```python
from build123d import *

# Parameters (mm, degrees)
BOSS_EXTRUDE1_DEPTH            = 4.4
BOSS_EXTRUDE2_START            = 4.4
BOSS_EXTRUDE2_DEPTH            = 40
BOSS_EXTRUDE3_START            = 4.4
BOSS_EXTRUDE3_DEPTH            = 3
CUT_EXTRUDE1_START             = -37
CUT_EXTRUDE1_DEPTH             = 37
CUT_EXTRUDE2_DEPTH             = 120.718001988
CUT_EXTRUDE2_DEPTH_BACK        = 120.718001988
FILLET1_R                      = 10
CUT_EXTRUDE3_REACH             = 121.718
CUT_EXTRUDE3_DIRECTION_2_REACH = 121.718
FILLET2_R                      = 1
CHAMFER1_SIZE                  = 5
CUT_EXTRUDE4_REACH             = 141.367
CUT_EXTRUDE4_END_RADIUS        = 65


with BuildPart() as part:
    # Sketch1 → Boss-Extrude1 (new body)
    with BuildSketch(Plane(origin=(0, 0, 0), x_dir=(1, 0, 0), z_dir=(0, 1, 0))):
        with BuildLine():
            Line((-31.320919527, 25.2), (31.320919527, 25.2))
            Line((31.320919527, 25.2), (51.0779796, 40.2))
            ThreePointArc((51.0779796, 40.2), (-65, 0), (51.0779796, -40.2))
            Line((51.0779796, -40.2), (31.320919527, -25.2))
            Line((31.320919527, -25.2), (-31.320919527, -25.2))
            ThreePointArc((-31.320919527, -25.2), (-40.2, 0), (-31.320919527, 25.2))
        make_face()
    extrude(amount=BOSS_EXTRUDE1_DEPTH)

    # Sketch1<3> → Boss-Extrude2 (add)
    with BuildSketch(Plane(origin=(0, 0, 0), x_dir=(1, 0, 0), z_dir=(0, 1, 0)).offset(BOSS_EXTRUDE2_START)):
        with BuildLine():
            ThreePointArc((0, -55), (-55, 0), (0, 55))
            Line((0, 55), (34.641016151, 55))
            ThreePointArc((34.641016151, 55), (-65, 0), (34.641016151, -55))
            Line((34.641016151, -55), (0, -55))
        make_face()
    extrude(amount=BOSS_EXTRUDE2_DEPTH)

    # Sketch1<4> → Boss-Extrude3 (add)
    with BuildSketch(Plane(origin=(0, 0, 0), x_dir=(1, 0, 0), z_dir=(0, 1, 0)).offset(BOSS_EXTRUDE3_START)):
        with BuildLine():
            ThreePointArc((-40.2, 0), (-37.915306704, 13.359248389), (-31.320919527, 25.2))
            ThreePointArc((-31.320919527, 25.2), (-17.363755354, 36.256585609), (0, 40.2))
            Line((0, 40.2), (37.536115942, 40.2))
            ThreePointArc((37.536115942, 40.2), (20.174241002, 51.166395222), (0, 55))
            ThreePointArc((0, 55), (-38.890872965, 38.890872965), (-55, 0))
            Line((-55, 0), (-40.2, 0))
        make_face()
        with BuildLine():
            ThreePointArc((-31.320919527, -25.2), (-37.915306704, -13.359248389), (-40.2, 0))
            Line((-40.2, 0), (-55, 0))
            ThreePointArc((-55, 0), (-38.890872965, -38.890872965), (0, -55))
            ThreePointArc((0, -55), (20.174241002, -51.166395222), (37.536115942, -40.2))
            Line((37.536115942, -40.2), (0, -40.2))
            ThreePointArc((0, -40.2), (-17.363755354, -36.256585609), (-31.320919527, -25.2))
        make_face()
        with BuildLine():
            ThreePointArc((37.536115942, -40.2), (20.174241002, -51.166395222), (0, -55))
            Line((0, -55), (34.641016151, -55))
            ThreePointArc((34.641016151, -55), (43.493638134, -48.304279747), (51.0779796, -40.2))
            Line((51.0779796, -40.2), (37.536115942, -40.2))
        make_face()
        with BuildLine():
            ThreePointArc((0, 55), (20.174241002, 51.166395222), (37.536115942, 40.2))
            Line((37.536115942, 40.2), (51.0779796, 40.2))
            ThreePointArc((51.0779796, 40.2), (43.493638134, 48.304279747), (34.641016151, 55))
            Line((34.641016151, 55), (0, 55))
        make_face()
    extrude(amount=BOSS_EXTRUDE3_DEPTH)

    # Sketch2 → Cut-Extrude1 (cut)
    with BuildSketch(Plane(origin=(0, 44.4, 0), x_dir=(1, 0, 0), z_dir=(0, 1, 0)).offset(CUT_EXTRUDE1_START)):
        with BuildLine():
            Line((-47.634201136, -27.495142883), (-55.300459871, -34.15931993))
            ThreePointArc((-55.300459871, -34.15931993), (-49.056122714, -42.643836884), (-41.523220262, -50.008221115))
            Line((-41.523220262, -50.008221115), (-33.856961527, -43.344044068))
            ThreePointArc((-33.856961527, -43.344044068), (-41.509026912, -36.083246594), (-47.634201136, -27.495142883))
        make_face()
        with BuildLine():
            Line((-33.856961527, -43.344044068), (-41.523220262, -50.008221115))
            Line((-41.523220262, -50.008221115), (-22.894930026, -50.008221115))
            ThreePointArc((-22.894930026, -50.008221115), (-28.570913752, -46.996839121), (-33.856961527, -43.344044068))
        make_face()
    extrude(amount=CUT_EXTRUDE1_DEPTH, mode=Mode.SUBTRACT)

    # Sketch3 → Cut-Extrude2 (cut, two sides: drawn at the far end of the back side and taken through both)
    with BuildSketch(Plane.XY.offset(-25.2).offset(-CUT_EXTRUDE2_DEPTH_BACK)):
        with BuildLine():
            Line((34.641016151, 44.4), (-25.358983849, 44.4))
            ThreePointArc((-25.358983849, 44.4), (9.372126125, 35.01047424), (34.641016151, 9.4))
            Line((34.641016151, 9.4), (34.641016151, 44.4))
        make_face()
    extrude(amount=CUT_EXTRUDE2_DEPTH + CUT_EXTRUDE2_DEPTH_BACK, mode=Mode.SUBTRACT)

    # Fillet1
    fillet1_edges = [part.edges().sort_by_distance(p)[0] for p in [
        (31.320919527, 2.2, -25.2),
        (31.320919527, 2.2, 25.2),
    ]]
    fillet(fillet1_edges, radius=FILLET1_R)

    # Cut-Extrude3: up to this face of the body (flat: up to its plane)
    cut_extrude3_end = Plane(part.part.faces().sort_by_distance((25.5389898, 5.9, -40.2))[0])
    # Sketch4 → Cut-Extrude3 (cut, up to the picked face)
    with BuildSketch(Plane.XY.offset(-25.2), mode=Mode.PRIVATE) as cut_extrude3_sk1:
        Polygon((51.0779796, 4.4), (27.954908691, 4.4), (51.0779796, 2.9), align=None)
    cut_extrude3_tool1 = split(extrude(cut_extrude3_sk1.sketch, amount=-CUT_EXTRUDE3_REACH, mode=Mode.PRIVATE), bisect_by=cut_extrude3_end, keep=Keep.BOTH, mode=Mode.PRIVATE)
    # Sketch4 → Cut-Extrude3 (cut, up to the picked face)
    with BuildSketch(Plane.XY.offset(-25.2), mode=Mode.PRIVATE) as cut_extrude3_sk2:
        Polygon((51.0779796, 0), (51.0779796, 1.5), (27.954908691, 0), align=None)
    cut_extrude3_tool2 = split(extrude(cut_extrude3_sk2.sketch, amount=-CUT_EXTRUDE3_REACH, mode=Mode.PRIVATE), bisect_by=cut_extrude3_end, keep=Keep.BOTH, mode=Mode.PRIVATE)
    add(cut_extrude3_tool1.solids().sort_by(Axis((43.370289, 3.9, -25.2), (0, 0, -1)))[0], mode=Mode.SUBTRACT)
    add(cut_extrude3_tool2.solids().sort_by(Axis((43.370289, 0.5, -25.2), (0, 0, -1)))[0], mode=Mode.SUBTRACT)

    # Cut-Extrude3 direction 2: up to this face of the body (flat: up to its plane)
    cut_extrude3_direction_2_end = Plane(part.part.faces().sort_by_distance((25.5389898, 5.9, 40.2))[0])
    # Sketch4 → Cut-Extrude3 direction 2 (cut, up to the picked face)
    with BuildSketch(Plane.XY.offset(-25.2), mode=Mode.PRIVATE) as cut_extrude3_direction_2_sk1:
        Polygon((51.0779796, 4.4), (27.954908691, 4.4), (51.0779796, 2.9), align=None)
    cut_extrude3_direction_2_tool1 = split(extrude(cut_extrude3_direction_2_sk1.sketch, amount=CUT_EXTRUDE3_DIRECTION_2_REACH, mode=Mode.PRIVATE), bisect_by=cut_extrude3_direction_2_end, keep=Keep.BOTH, mode=Mode.PRIVATE)
    # Sketch4 → Cut-Extrude3 direction 2 (cut, up to the picked face)
    with BuildSketch(Plane.XY.offset(-25.2), mode=Mode.PRIVATE) as cut_extrude3_direction_2_sk2:
        Polygon((51.0779796, 0), (51.0779796, 1.5), (27.954908691, 0), align=None)
    cut_extrude3_direction_2_tool2 = split(extrude(cut_extrude3_direction_2_sk2.sketch, amount=CUT_EXTRUDE3_DIRECTION_2_REACH, mode=Mode.PRIVATE), bisect_by=cut_extrude3_direction_2_end, keep=Keep.BOTH, mode=Mode.PRIVATE)
    add(cut_extrude3_direction_2_tool1.solids().sort_by(Axis((43.370289, 3.9, -25.2), (0, 0, 1)))[0], mode=Mode.SUBTRACT)
    add(cut_extrude3_direction_2_tool2.solids().sort_by(Axis((43.370289, 0.5, -25.2), (0, 0, 1)))[0], mode=Mode.SUBTRACT)

    # Fillet2
    fillet2_edges = [part.edges().sort_by_distance(p)[0] for p in [
        (-41.523220262, 25.9, 50.008221115),
    ]]
    fillet(fillet2_edges, radius=FILLET2_R)

    # Chamfer1
    chamfer1_edges = [part.edges().sort_by_distance(p)[0] for p in [
        (-51.467330503, 44.4, 30.827231407),
    ]]
    chamfer(chamfer1_edges, length=CHAMFER1_SIZE)

    # Cut-Extrude4: up to this cylinder (the profile starts inside it)
    cut_extrude4_end = Plane(origin=(0, 42.733333, 0), z_dir=(0, -1, 0)) * Cylinder(CUT_EXTRUDE4_END_RADIUS, 413.734, mode=Mode.PRIVATE)
    # Sketch5 → Cut-Extrude4 (cut, up to the surface)
    with BuildSketch(Plane(origin=(0, 0, 50.008221115), x_dir=(-1, 0, 0), z_dir=(0, 0, -1)), mode=Mode.PRIVATE) as cut_extrude4_sk1:
        Polygon((34.654383693, 44.4), (39.654383693, 39.4), (39.654383693, 44.4), align=None)
    cut_extrude4_tool1 = extrude(cut_extrude4_sk1.sketch, amount=-CUT_EXTRUDE4_REACH, mode=Mode.PRIVATE) & cut_extrude4_end
    add(cut_extrude4_tool1.solids().sort_by_distance((-37.987717, 42.733333, 50.008221))[0], mode=Mode.SUBTRACT)


solid = part.part
```
Input: part model. Units: mm. Frame: model coordinates. A direction names the side the tool comes from. Give positions to 0.01 mm unless a question says otherwise; leave off trailing zeros. Order: outer loops, then holes, each group sorted by start corner. A loop starts at its lowest first (then second) coordinate and runs counter-clockwise, first axis right, second up. Notation, with made-up numbers: (35.25, 17) - (53.25, 17) arc R25 ccw to (53.25, 38) - close; hole circle Ø11 at (77.25, 20). An arc over 180 degrees is marked (long way). One line per item, written item: value.
1. Pin query (flat end, axial travel): pin 1 Ø1.2 at (x, y) = (34.5, 1) entering from -Z; pin 2 Ø10 at (y, z) = (20.5, 35) entering from +X; pin 3 Ø3 at (y, z) = (6.5, 29.5) entering from -X. Return the tip coordinate at first contact, or that it passes through.
Determined:
pin 1: z = -55.46
pin 2: x = -50.52
pin 3: x = -58.66
2. Cut plane A-A, the plane x = 40.5. Output: boundary loops of the cut face in (y, z).
Determined:
outline: (0, -50.84) - (7.4, -50.84) - (7.4, -40.2) - (3.59, -40.2) - (3.59, -32.17) - (0.81, -32.17) - (0.81, -40.2) - (0, -40.2) - close; (0, 40.2) - (0.81, 40.2) - (0.81, 32.17) - (3.59, 32.17) - (3.59, 40.2) - (7.4, 40.2) - (7.4, 50.84) - (0, 50.84) - close
3. Cut plane D-D, the plane x = -17. Output: boundary loops of the cut face in (y, z).
Determined:
outline: (0, -62.74) - (43.89, -62.74) - (43.89, -52.31) - (7.4, -52.31) - (7.4, -36.43) - (4.4, -36.43) - (4.4, -25.2) - (0, -25.2) - close; (0, 25.2) - (4.4, 25.2) - (4.4, 36.43) - (7.4, 36.43) - (7.4, 52.31) - (43.89, 52.31) - (43.89, 62.74) - (0, 62.74) - close
4. Cut plane C-C, the plane z = -18. Output: boundary loops of the cut face in (x, y).
Determined:
outline: (-62.46, 0) - (-35.94, 0) - (-35.94, 7.4) - (-51.97, 7.4) - (-51.97, 44.4) - (-62.46, 44.4) - close
5. Reachability of faces 1 (the face through (31.102, 2.231, -25.708)), 2 (the face through (-51.41, 23.18, 30.78)), 3 (the face through (37.109, 0.594, 34.262)), 4 (the face through (14, 20, 55)) from +Z, -Z, +X, -X, +Y, -Y: full face, straight path, thin tool, end or side. Return the list, or none.
Determined:
face 1: +X, +Y, -Y
face 2: +Z, +X, +Y
face 3: +X, -Y
face 4: +X, +Y
6. Line query: probe 1 along Y at (x, z) = (-41, -29); probe 2 along Y at (x, z) = (15, 29); probe 3 along Z at (x, y) = (19.5, 3.5). Output: solid intervals per line, ascending.
Determined:
probe 1: 0 to 7.4
probe 2: 0 to 4.4
probe 3: -62.01 to -25.2, 25.2 to 62.01
7. Cut plane B-B, the plane y = 23. Output: boundary loops of the cut face in (x, z).
Determined:
outline: (-55.3, 34.16) arc R65 ccw to (24.56, -60.18) - (24.56, -55) - (0, -55) arc R55 cw to (-47.63, 27.5) - close; (-39.26, 51.81) arc R1 ccw to (-38.65, 50.01) - (-22.89, 50.01) arc R55 cw to (0, 55) - (24.56, 55) - (24.56, 60.18) arc R65 ccw to start
